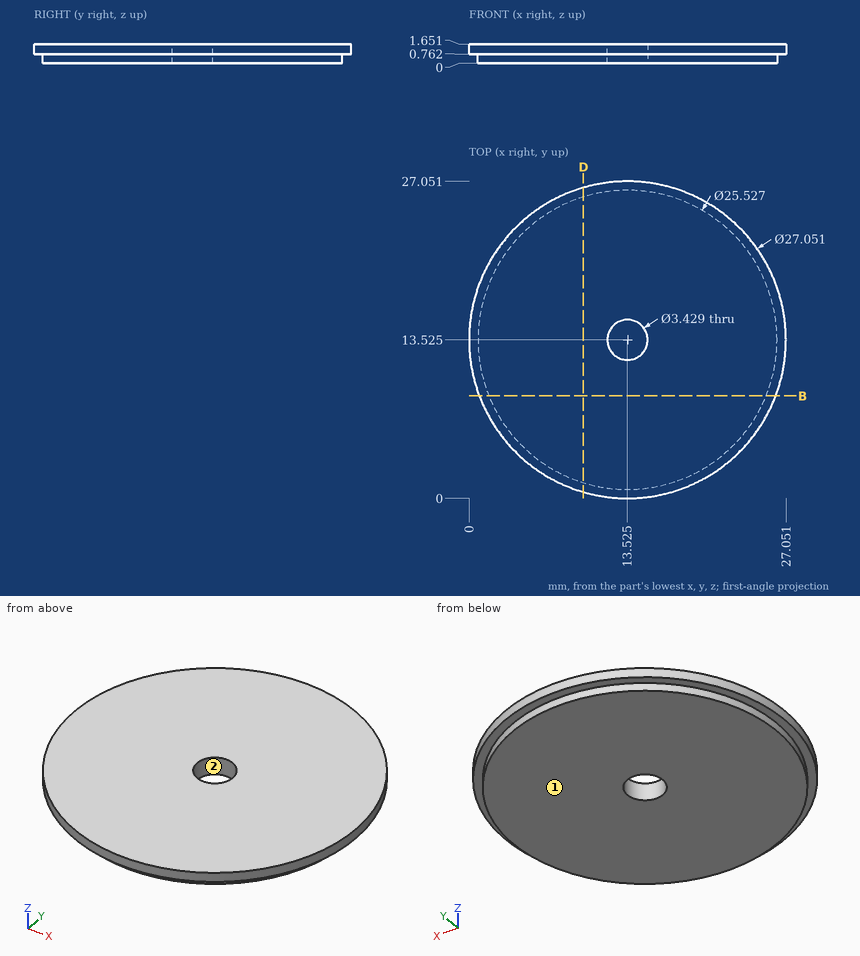
Geometry: see drawing. Coordinates: mm, zero at the bounding-box minimum. Coordinates: 2 decimals unless noted, no trailing zeros. Loops run counter-clockwise (first coordinate to the right, second up) from the corner with the lowest first, then second, coordinate; pieces in that order, holes last. Notation, with made-up numbers: M 48,64.25 L 67,64.25 A24 cw 67,103.25 Z; hole C 6.5,28 d6. An arc over 180 degrees is marked long. Answer in a Markdown table with one row per item.
Q1. Section D-D on x = 9.75. Return the cut outline in (y, z).
Answers below:
| item | result |
|---|---|
| outline | M 0.54,0.76 L 1.33,0.76 L 1.33,0 L 25.72,0 L 25.72,0.76 L 26.51,0.76 L 26.51,1.65 L 0.54,1.65 Z |
Q2. First-contact query: pin 1 (2 mm diameter, centred on x = 5.5, y = 10.5, fed in from -Z). Flat tip, straight axial feed; report the tip coordinate or a pass-through.
Answers below:
| item | result |
|---|---|
| pin 1 | stops at z = 0 |
Q3. Ray query, probe 1 along X at (y, z) = (13.5, 1.15); probe 2 along Y at (x, z) = (17.5, 0.45) (1 decimal); probe 3 along X at (y, z) = (19.25, 0.65) (1 decimal). Return the intervals inside material, ascending. Write a range as from..to.
Answers below:
| item | result |
|---|---|
| probe 1 | x = 0..11.81, 15.24..27.05 |
| probe 2 | y = 1.4..25.7 |
| probe 3 | x = 2.1..24.9 |
Q4. Draft query along X for the marked faces 1 and 2. Return one class per face: pulls with the +X half, pulls with the -X half, needs draft (parallel to the pull), parting line crosses it, or undercut.
Answers below:
| item | result |
|---|---|
| face 1 | needs draft |
| face 2 | undercut |
Q5. Section B-B on y = 8.75. Return the cut outline in (x, z).
Answers below:
| item | result |
|---|---|
| outline | M 0.87,0.76 L 1.69,0.76 L 1.69,0 L 25.36,0 L 25.36,0.76 L 26.18,0.76 L 26.18,1.65 L 0.87,1.65 Z |
